Check sheet for the modelled part. Datum: model origin and axes. Units: mm. Face numbers are marked on the shaded views. A direction names the side the tool comes from. Give positions to 0.01 mm unless a question says otherwise; leave off trailing zeros. Write each loop counter-clockwise with the first axis right and the second up, starting at its lowest first coordinate (ties: lowest second). Pieces come first, ordered by that corner, then holes. Notation, with made-up numbers: (-27.5, -18) -> (10.5, -18) arc R34 cw to (10.5, 17) -> close; hole circle Ø2 at (60.5, 52). An arc over 180 degrees is marked (long way). Return JSON: item names as keys, results as strings.
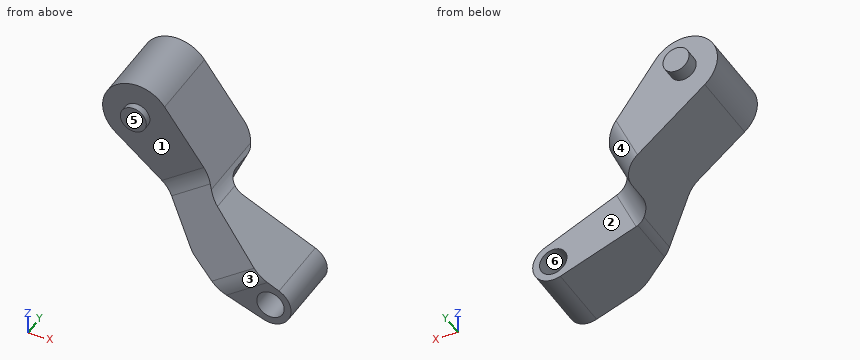
from build123d import *

# Parameters (mm, degrees)
F0_R          = 10
F0_R_2        = 9.5
F1_DEPTH      = 95
F3_DEPTH      = 103.0741500701
F3_DEPTH_BACK = 97.783322066
F4_W          = 111.3981074931
F4_H          = 45
F5_DEPTH      = 88.2146892838
F5_DEPTH_BACK = 25
F6_R          = 15
F7_R          = 20
F8_R          = 9.5
F9_DEPTH      = 5
F9_DEPTH_BACK = 65
F10_R         = 20


with BuildPart() as f1:
    # F0 (on Front) → F1 (new body)
    with BuildSketch(Plane.XZ):
        with BuildLine():
            Line((40.472202318, 47.836435473), (0.5161550447, 102.8184539019))
            ThreePointArc((0.5161550447, 102.8184539019), (-36.9259098509, 106.247026954), (-35.422653502, 68.6783756984))
            Line((-35.422653502, 68.6783756984), (34.0419716339, 12.5334943419))
            Line((34.0419716339, 12.5334943419), (93.7381570012, -9.3650366096))
            ThreePointArc((93.7381570012, -9.3650366096), (112.7797489078, -0.9804332321), (105.1254790408, 18.3662964382))
            Line((105.1254790408, 18.3662964382), (40.472202318, 47.836435473))
        make_face()
        with Locations((98.9040414947, 4.7173508797)):
            Circle(F0_R, mode=Mode.SUBTRACT)
        with Locations((-19.7076478051, 88.121590349)):
            Circle(F0_R_2, mode=Mode.SUBTRACT)
    extrude(amount=F1_DEPTH)

    # F2 (on face) → F3 (cut, two sides)
    with BuildSketch(Plane(origin=(49.2343596113, 0, 35.7791593745), x_dir=(0, 1, 0), z_dir=(0.808952114, 0, 0.5878745421))) as f3_sk:
        Polygon((-55, 28.273306787), (-55, 107.9234746602), (-95, 107.9234746602), (-95, -12.0765253398), (-95, -32.8742563725), align=None)
    extrude(amount=-F3_DEPTH, mode=Mode.SUBTRACT)
    extrude(f3_sk.sketch, amount=F3_DEPTH_BACK, mode=Mode.SUBTRACT)

    # F4 (on face) → F5 (cut, two sides)
    with BuildSketch(Plane(origin=(25.0160459603, 0, 54.8816325595), x_dir=(0.9099297039, 0, -0.4147625031), z_dir=(0.4147625031, 0, 0.9099297039))) as f5_sk:
        with Locations((71.1682909773, -22.5)):
            Rectangle(F4_W, F4_H)
    extrude(amount=-F5_DEPTH, mode=Mode.SUBTRACT)
    extrude(f5_sk.sketch, amount=F5_DEPTH_BACK, mode=Mode.SUBTRACT)

    # F6
    f6_edges = [f1.edges().sort_by_distance(p)[0] for p in [
        (32.605588, -45, 34.23539),
        (32.605588, 0, 34.23539),
    ]]
    fillet(f6_edges, radius=F6_R)

    # F7
    f7_edges = [f1.edges().sort_by_distance(p)[0] for p in [
        (40.472202, -50.159062, 47.836435),
        (34.041972, -62.100604, 12.533494),
    ]]
    fillet(f7_edges, radius=F7_R)

    # F8 (on face) → F9 (join, two sides)
    with BuildSketch(Plane.XZ.offset(55)) as f9_sk:
        with Locations((-19.7076478051, 88.121590349)):
            Circle(F8_R)
    extrude(amount=F9_DEPTH)
    extrude(f9_sk.sketch, amount=-F9_DEPTH_BACK)

    # F10
    f10_edges = [f1.edges().sort_by_distance(p)[0] for p in [
        (17.967044, -55, 48.007383),
        (75.23055, -95, 14.032807),
    ]]
    fillet(f10_edges, radius=F10_R)


solid = f1.part
(1) Cross-section at B-B on z = 82.5. Enter the section's corners in (x, y), then the cut area to 3 significant figures.
Reply:
{"outline": "(-44.07, -55) -> (-27.37, -55) -> (-27.37, -60) -> (-12.05, -60) -> (-12.05, -55) -> (15.28, -55) -> (15.28, 0) -> (-12.05, 0) -> (-12.05, 10) -> (-27.37, 10) -> (-27.37, 0) -> (-44.07, 0) -> close", "area": "3,490 mm^2"}
(2) Thickness scan on L1, parallel to Y at x = 22, z = 58; L2, parallel to Y at x = -24, z = 90; L3, parallel to Z at x = 18, y = -61. Record the ranges inside material, lowest first.
Reply:
{"L1": "-55 to 0", "L2": "-60 to 10", "L3": "25.5 to 36.69"}
(3) Cross-section at D-D on x = -8. Enter the section's corners in (y, z), then the cut area to 3 significant figures.
Reply:
{"outline": "(-55, 46.51) -> (0, 46.51) -> (0, 110.21) -> (-55, 110.21) -> close", "area": "3,500 mm^2"}
(4) Cross-section at C-C on y = -88. Enter the section's corners in (x, z).
Reply:
{"outline": "(47.95, 7.43) -> (93.74, -9.37) arc R15 ccw to (105.13, 18.37) -> (79.23, 30.17) -> close; hole circle Ø20 at (98.9, 4.72)"}
(5) Set-up check for the marked faces 1, 2 and 3: record each of +Z, -Z, +X, -X, +Y, -Y from which the full face is reachable in a straight line by a thin tool's end or side.
Reply:
{"face 1": "-Y", "face 2": "-Z, +X, +Y", "face 3": "+Z, -X, -Y"}
(6) Release check for a two-part mould opening along X. For the marked faces 4, 5 and 6 record: pulls with the +X half, pulls with the -X half, needs draft (parallel to the pull), parting line crosses it, or undercut.
Reply:
{"face 4": "pulls with the +X half", "face 5": "needs draft", "face 6": "undercut"}
(7) Cross-section at A-A on y = -72. Enter the section's corners in (x, z), then the cut area to 3 significant figures.
Reply:
{"outline": "(24.25, 20.45) -> (31.47, 14.62) arc R20 ccw to (37.15, 11.39) -> (93.74, -9.37) arc R15 ccw to (105.13, 18.37) -> (53.66, 41.82) -> close; hole circle Ø20 at (98.9, 4.72)", "area": "2,180 mm^2"}
(8) Depth check by flat-ended pin: pin 1 Ø16 at (x, z) = (78.5, 18.5) entering from +Y; pin 2 Ø1 at (y, z) = (-74, 43) entering from -X; pin 3 Ø21 at (x, z) = (-20.5, 92) entering from -Y. Enter the tip coordinate at first touch or a pass-through.
Reply:
{"pin 1": "y = -45", "pin 2": "through", "pin 3": "y = -60"}
